from build123d import *

# Parameters (mm, degrees)
F3_START = -7.62
F2_R     = 4.826
F3_DEPTH = 93.981


with BuildPart() as f1:
    # F0 (on Front) → F1 (revolve)
    with BuildSketch(Plane.XZ):
        with BuildLine():
            Line((0, 3.175), (0, 7.1581820314))
            Line((0, 7.1581820314), (0, 12.7))
            Line((0, 12.7), (-6.35, 12.7))
            Line((-6.35, 12.7), (-6.35, 9.6808019567))
            ThreePointArc((-6.35, 9.6808019567), (-7.2573194714, 7.7350490712), (-9.3310663713, 7.179390264))
            Line((-9.3310663713, 7.179390264), (-40.64, 12.7))
            Line((-40.64, 12.7), (-99.4210244843, 12.7))
            ThreePointArc((-99.4210244843, 12.7), (-101.0513051228, 6.4427853895), (-101.6, 0))
            Line((-101.6, 0), (-40.64, 0))
            Line((-40.64, 0), (-40.64, 3.175))
            Line((-40.64, 3.175), (0, 3.175))
        make_face()
    revolve(axis=Axis((-71.12, 0, 0), (1, 0, 0)))

    # F2 (on face) → F3 (cut)
    with BuildSketch(Plane.YZ.offset(F3_START)):
        with Locations((-14.1259352998, -7.4992162652)):
            Circle(F2_R)
        with Locations((-13.557479444, 8.4838106893)):
            Circle(F2_R)
        with Locations((0.5684558558, 15.9830269545)):
            Circle(F2_R)
        with Locations((14.1259352998, 7.4992162652)):
            Circle(F2_R)
        with Locations((13.557479444, -8.4838106893)):
            Circle(F2_R)
        with Locations((-0.5684558558, -15.9830269545)):
            Circle(F2_R)
    extrude(amount=-F3_DEPTH, mode=Mode.SUBTRACT)


solid = f1.part
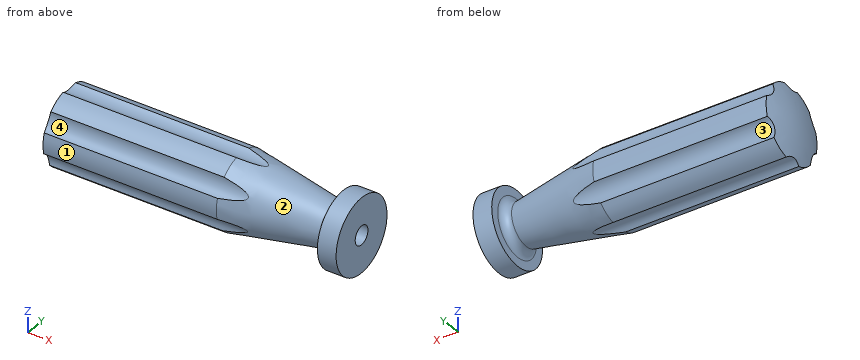
Input: part model. Units: mm. Frame: model coordinates. Face numbers are marked on the shaded views. A direction names the side the tool comes from. Coordinates: 2 decimals unless noted, no trailing zeros. Order: outer loops, then holes, each group sorted by start corner. A loop starts at its lowest first (then second) coordinate and runs counter-clockwise, first axis right, second up. Notation, with made-up numbers: M -6.5,8 L 32.5,8 A27 cw 32.5,35 Z; hole C 44,-13 d6. An arc over 180 degrees is marked long. Answer in a Markdown table with one row per item.
(1) Section query A-A, the plane x = -82. Output: boundary loops of the cut face in (y, z), plus the area to 3 significant figures.
Numbers:
| item | result |
|---|---|
| outline | M -12.34,-3.02 A4.83 cw -9.41,-8.53 A12.7 ccw -3.56,-12.19 A4.83 cw 2.68,-12.41 A12.7 ccw 8.78,-9.17 A4.83 cw 12.09,-3.89 A12.7 ccw 12.34,3.02 A4.83 cw 9.41,8.53 A12.7 ccw 3.56,12.19 A4.83 cw -2.68,12.41 A12.7 ccw -8.78,9.17 A4.83 cw -12.09,3.89 A12.7 ccw Z |
| area | 468 mm^2 |
(2) Access query for the marked faces 1, 2, 3 and 4. Directions: +Z, -Z, +X, -X, +Y, -Y. A direction counts if a zero-diameter tool reaches every point of the face in a straight line with its end or side. Return the directions, or none.
Numbers:
| item | result |
|---|---|
| face 1 | +X, -X, -Y |
| face 2 | none |
| face 3 | -X, +Y |
| face 4 | -X, -Y |
(3) Contact query for flat-ended pins moving along their axis: pin 1 Ø1.9 at (y, z) = (0.5, -1) entering from +X; pin 2 Ø1 at (x, z) = (-78.5, 2.5) entering from -Y; pin 3 Ø10 at (y, z) = (-8, 2.5) entering from -X. Output: stop coordinate, or through.
Numbers:
| item | result |
|---|---|
| pin 1 | stops at x = -40.64 |
| pin 2 | stops at y = -12.54 |
| pin 3 | stops at x = -101.45 |
(4) Section query C-C, the plane z = 0. Output: boundary loops of the cut face in (x, y) (3 decimals), plus the area to 3 significant figures.
Numbers:
| item | result |
|---|---|
| outline | M -99.421,-12.7 L -40.64,-12.7 L -9.331,-7.179 A2.54 cw -6.35,-9.681 L -6.35,-12.7 L 0,-12.7 L 0,-3.175 L -40.64,-3.175 L -40.64,3.175 L 0,3.175 L 0,12.7 L -6.35,12.7 L -6.35,9.681 A2.54 cw -9.331,7.179 L -40.64,12.7 L -99.421,12.7 A38.1 ccw Z |
| area | 2,100 mm^2 |
(5) Section query D-D, the plane x = -20. Output: boundary loops of the cut face in (y, z) (3 decimals), plus the area to 3 significant figures.
Numbers:
| item | result |
|---|---|
| outline | C 0,0 d18.121; hole C 0,0 d6.35 |
| area | 226 mm^2 |
(6) Material intervals for line 1 (Z direction, x = -23.5, y = 0) (3 decimals); line 2 (Y direction, x = -15.5, z = -0.5); line 3 (Y direction, x = -16.5, z = 0) (3 decimals), sorted ascending. Write a range as [from, to].
Numbers:
| item | result |
|---|---|
| line 1 | z = [-9.678, -3.175], [3.175, 9.678] |
| line 2 | y = [-8.25, -3.14], [3.14, 8.25] |
| line 3 | y = [-8.443, -3.175], [3.175, 8.443] |
